Check sheet for the modelled part. Datum: model origin and axes. Units: mm. A direction names the side the tool comes from. Give positions to 0.01 mm unless a question says otherwise; leave off trailing zeros. Write each loop counter-clockwise with the first axis right and the second up, starting at its lowest first coordinate (ties: lowest second). Pieces come first, ordered by that corner, then holes. Notation, with made-up numbers: (-24, 4) -> (4, 4) arc R26 cw to (4, 28) -> close; hole circle Ø3 at (78.25, -16.75). An arc over 180 degrees is marked (long way). Return JSON: item names as keys, results as strings.
from build123d import *

# Parameters (mm, degrees)
ESQUISSE1_R        = 7.5
ESQUISSE1_R_2      = 4
BOSS_EXTRU_1_DEPTH = 12
ESQUISSE4_W        = 1
ESQUISSE4_H        = 1
ESQUISSE6_W        = 1.6
ESQUISSE6_H        = 1.2


with BuildPart() as part:
    # Esquisse1 → Boss.-Extru.1 (new body)
    with BuildSketch(Plane(origin=(0, 0, 0), x_dir=(1, 0, 0), z_dir=(0, 1, 0))):
        Circle(ESQUISSE1_R)
        Circle(ESQUISSE1_R_2, mode=Mode.SUBTRACT)
    extrude(amount=BOSS_EXTRU_1_DEPTH)

    # Enlèvement de matière-Balayage1: sweep along a path in Esquisse2
    with BuildLine(Plane(origin=(0, 4, 0), x_dir=(-1, 0, 0), z_dir=(0, -1, 0))) as enl_vement_de_mati_re_balayage1_path:
        CenterArc((0, 0), 7.5, 0, 360)
    # Esquisse4 → Enlèvement de matière-Balayage1 (sweep, cut)
    with BuildSketch(Plane.XY):
        with Locations((-7.5, 4)):
            Rectangle(ESQUISSE4_W, ESQUISSE4_H)
    sweep(path=enl_vement_de_mati_re_balayage1_path.line, mode=Mode.SUBTRACT)

    # Enlèvement de matière-Balayage2: sweep along a path in Esquisse5
    with BuildLine(Plane(origin=(0, 0, 0), x_dir=(-1, 0, 0), z_dir=(0, -1, 0))) as enl_vement_de_mati_re_balayage2_path:
        CenterArc((0, 0), 5.75, 0, 360)
    # Esquisse6 → Enlèvement de matière-Balayage2 (sweep, cut)
    with BuildSketch(Plane(origin=(0, 0, 0), x_dir=(0, 0, -1), z_dir=(1, 0, 0))):
        with Locations((5.75, 0)):
            Rectangle(ESQUISSE6_W, ESQUISSE6_H)
    sweep(path=enl_vement_de_mati_re_balayage2_path.line, mode=Mode.SUBTRACT)

    # Symétrie1: part across plane


with BuildPart() as part_1:
    add(part.part)
    add(part.part.mirror(Plane.ZX.offset(12)))


solid = part_1.part
(1) Set-up check for faces 5 (the cylindrical face through (-4.72, 0.3, -1.49)), 6 (the cylindrical face through (-6.466, 4.007, 2.681)), 7 (the cylindrical face through (-4.72, 23.7, -1.49)), 8 (the flat face through (2, 0, 4)), 9 (the cylindrical face through (-0.867, 12.168, 3.905)): record each of +Z, -Z, +X, -X, +Y, -Y from which the full face is reachable in a straight line by a thin tool's end or side.
Reply:
{"face 5": "-Y", "face 6": "none", "face 7": "+Y", "face 8": "+Z, -Z, +X, -X, -Y", "face 9": "+Y, -Y"}
(2) Depth check by flat-ended pin: pin 1 Ø1 at (x, y) = (5.5, 11) entering from -Z; pin 2 Ø6 at (x, y) = (3.5, 9.5) entering from +Z; pin 3 Ø1.5 at (y, z) = (6, 1.5) entering from -X. Enter the tip coordinate at first touch or a pass-through.
Reply:
{"pin 1": "z = -5.59", "pin 2": "z = 7.48", "pin 3": "x = -7.46"}
(3) Cross-section at A-A on y = 5.5. Enter the section's corners in (x, z).
Reply:
{"outline": "circle Ø15 at (0, 0); hole circle Ø8 at (0, 0)"}
(4) Release check for a two-part mould opening along Y. For faces 1 (the flat face through (2, 24, 4)), 2 (the cylindrical face through (-3.521, 23.696, -5.523)), 3 (the flat face through (0, 0, 7)), 4 (the cylindrical face through (-6.466, 19.993, 2.681)) record: pulls with the +Y half, pulls with the -Y half, needs draft (parallel to the pull), parting line crosses it, or undercut.
Reply:
{"face 1": "pulls with the +Y half", "face 2": "needs draft", "face 3": "pulls with the -Y half", "face 4": "undercut"}
(5) Thickness scan on L1, parallel to Y at x = 4.25, z = -5.75; L2, parallel to X at y = 0.45, z = 0. Record the ranges inside material, lowest first.
Reply:
{"L1": "0 to 3.5, 4.5 to 19.5, 20.5 to 24", "L2": "-7.5 to -6.55, -4.95 to -4, 4 to 4.95, 6.55 to 7.5"}
